```python
from build123d import *

# Parameters (mm, degrees)
SKETCH_1_W          = 8
SKETCH_1_H          = 21.4
EXTRUDE_1_DEPTH     = 15.7
CUT_EXTRUDE_START   = 15.7
SKETCH_1_18_R       = 2.6
CUT_EXTRUDE_1_DEPTH = 2.6
SKETCH_2_R          = 1.05
CUT_EXTRUDE_2_DEPTH = 23.443261795
SKETCH_3_R          = 2
CUT_EXTRUDE_4_DEPTH = 6
SKETCH_3_4_R        = 1.5
CUT_EXTRUDE_5_DEPTH = 23.443261795
SKETCH_4_R          = 0.8
CUT_EXTRUDE_6_DEPTH = 4
SKETCH_5_W          = 20.288493166
SKETCH_5_H          = 31.298439213
CUT_EXTRUDE_7_DEPTH = 30.490676493


with BuildPart() as part:
    # 草图1 → 凸台-拉伸1 (new body)
    with BuildSketch(Plane(origin=(0, 0, 0), x_dir=(1, 0, 0), z_dir=(0, 1, 0))):
        with Locations((0, -3.2)):
            Rectangle(SKETCH_1_W, SKETCH_1_H)
    extrude(amount=EXTRUDE_1_DEPTH)

    # 草图1<18> → 切除-拉伸1 (cut)
    with BuildSketch(Plane(origin=(0, 0, 0), x_dir=(1, 0, 0), z_dir=(0, 1, 0)).offset(CUT_EXTRUDE_START)):
        with Locations(Location((0, 0, 0), (0, 0, 90))):
            Circle(SKETCH_1_18_R)
    extrude(amount=-CUT_EXTRUDE_1_DEPTH, mode=Mode.SUBTRACT)

    # 草图2 → 切除-拉伸2 (cut, through all)
    with BuildSketch(Plane.ZY.offset(4)):
        with Locations((4.646826988, 10.35029737)):
            Circle(SKETCH_2_R)
    extrude(amount=-CUT_EXTRUDE_2_DEPTH, mode=Mode.SUBTRACT)

    # 草图3 → 切除-拉伸4 (cut)
    with BuildSketch(Plane(origin=(4, 0, 0), x_dir=(0, 0, -1), z_dir=(1, 0, 0))):
        with Locations((4.5, 2.5)):
            Circle(SKETCH_3_R)
        with Locations((-11.4, 2.5)):
            Circle(SKETCH_3_R)
    extrude(amount=-CUT_EXTRUDE_4_DEPTH, mode=Mode.SUBTRACT)

    # 草图3<4> → 切除-拉伸5 (cut, through all)
    with BuildSketch(Plane(origin=(4, 0, 0), x_dir=(0, 0, -1), z_dir=(1, 0, 0))):
        with Locations((4.5, 2.5)):
            Circle(SKETCH_3_4_R)
        with Locations((-11.4, 2.5)):
            Circle(SKETCH_3_4_R)
    extrude(amount=-CUT_EXTRUDE_5_DEPTH, mode=Mode.SUBTRACT)

    # 草图4 → 切除-拉伸6 (cut)
    with BuildSketch(Plane(origin=(4, 0, 0), x_dir=(0, 0, -1), z_dir=(1, 0, 0))):
        with Locations((-0.5, 4)):
            Circle(SKETCH_4_R)
        with Locations((-9.9, 12.7)):
            Circle(SKETCH_4_R)
    extrude(amount=-CUT_EXTRUDE_6_DEPTH, mode=Mode.SUBTRACT)


with BuildPart() as body_2:
    # 镜向1: mirrored copy
    add(part.part.mirror(Plane.ZX.offset(-10)))


with BuildPart() as part_1:
    add(part.part)

    # 草图5 → 切除-拉伸7 (cut, through all)
    with BuildSketch(Plane(origin=(0, -10, 0), x_dir=(1, 0, 0), z_dir=(0, 1, 0))):
        with Locations((1.793447893, -5.785280747)):
            Rectangle(SKETCH_5_W, SKETCH_5_H)
    extrude(amount=CUT_EXTRUDE_7_DEPTH, mode=Mode.SUBTRACT)


solid = body_2.part
```
Verification items for the finished model (mm, model axes). A direction names the side the tool comes from. Give positions to 0.01 mm unless a question says otherwise; leave off trailing zeros. Loops run counter-clockwise (first coordinate to the right, second up) from the corner with the lowest first, then second, coordinate; pieces in that order, holes last.
1. Section check A-A, the plane z = 11.4. Enter the section's corners in (x, y), then the cut area to 3 significant figures.
2. Section check D-D, the plane y = -32.7. Enter the section's corners in (x, z), then the cut area to 3 significant figures.
3. Mould release check, pull along Z, two halves, no side actions. Record for faces 4 (the cylindrical face through (-2.986, -23.987, -4.305)), 5 (the flat face through (0, -28, -7.5)), 6 (the flat face through (0, -28, 13.9)): released by +Z, released by -Z, zero draft, split by the parting line, or undercut.
4. Thickness scan on line 1 (Z direction, x = 1.5, y = -22.5); line 2 (Z direction, x = -2.5, y = -21.75); line 3 (Y direction, x = 1.1, z = 0.5). Record the ranges inside material, lowest first.
5. Section check B-B, the plane y = -22.5. Enter the section's corners in (x, z).
6. Set-up check for faces 1 (the flat face through (0, -35.7, 3)), 2 (the cylindrical face through (2.03, -31.99, 9.53)), 3 (the flat face through (0, -33.1, 0)): record each of +Z, -Z, +X, -X, +Y, -Y from which the full face is reachable in a straight line by a thin tool's end or side.
7. Section check C-C, the plane x = 3. Enter the section's corners in (y, z).
8. Go/stop test with flat-tipped pins: pin 1 Ø1.2 at (y, z) = (-23, 10.5) entering from +X; pin 2 Ø2.5 at (x, z) = (0.5, -0.5) entering from -Y; pin 3 Ø1.8 at (y, z) = (-24, 0.5) entering from +X; pin 4 Ø2.5 at (y, z) = (-22.5, 11.4) entering from -X. Record where each tip stops, or that it passes through.
Geometry says:
1. outline: (-4, -35.7) - (4, -35.7) - (4, -24.5) - (-2, -24.5) - (-2, -24) - (-4, -24) - close; (-4, -21) - (-2, -21) - (-2, -20.5) - (4, -20.5) - (4, -20) - (-4, -20) - close
1. area: 95.6 mm2
2. outline: (-4, -7.5) - (4, -7.5) - (4, 9.1) - (0, 9.1) - (0, 10.7) - (4, 10.7) - (4, 13.9) - (-4, 13.9) - close
2. area: 165 mm2
3. face 4: undercut
3. face 5: released by -Z
3. face 6: released by +Z
4. line 1: z = -7.5 to -6.5, -2.5 to 9.4, 13.4 to 13.9
4. line 2: z = -7.5 to -5.8, -3.2 to 10.1, 12.7 to 13.9
4. line 3: y = -33.1 to -24.8, -23.2 to -20
5. outline: (-4, -7.5) - (4, -7.5) - (4, -6.5) - (-2, -6.5) - (-2, -6) - (-4, -6) - close; (-4, -3) - (-2, -3) - (-2, -2.5) - (4, -2.5) - (4, 9.4) - (-2, 9.4) - (-2, 9.9) - (-4, 9.9) - close; (-4, 12.9) - (-2, 12.9) - (-2, 13.4) - (4, 13.4) - (4, 13.9) - (-4, 13.9) - close
6. face 1: +Z, -Z, +X, -X, -Y
6. face 2: +X
6. face 3: -Y
7. outline: (-35.7, -7.5) - (-20, -7.5) - (-20, 13.9) - (-35.7, 13.9) - close; hole circle Ø1.6 at (-32.7, 9.9); hole circle Ø2.1 at (-30.35, 4.65); hole circle Ø1.6 at (-24, 0.5); hole circle Ø4 at (-22.5, -4.5); hole circle Ø4 at (-22.5, 11.4)
8. pin 1: stops at x = -2
8. pin 2: stops at y = -33.1
8. pin 3: stops at x = 4
8. pin 4: passes through
